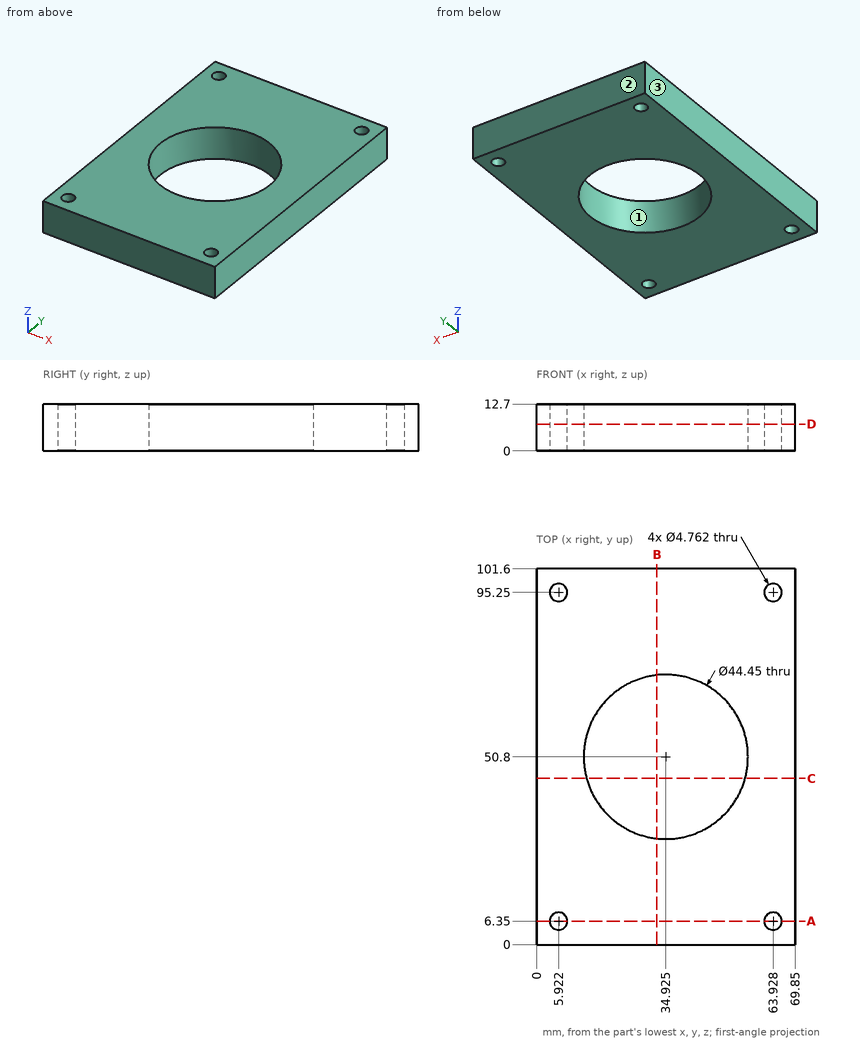
Source: three-view drawing plus pictorial views. Frame: mm from the lowest corner of the part. Coordinates: 2 decimals unless noted, no trailing zeros. Loops run counter-clockwise (first coordinate to the right, second up) from the corner with the lowest first, then second, coordinate; pieces in that order, holes last. Notation, with made-up numbers: (-14, 14.25) -> (14, 14.25) arc R25 cw to (14, 45.25) -> close; hole circle Ø8 at (83, 45). An arc over 180 degrees is marked (long way). One line per item, written item: value.
(1) Ray query, line 1 along Y through (x, z) = (4.5, 6.75); line 2 along Y through (x, z) = (63.5, 5.5); line 3 along Y through (x, z) = (26.5, 10) (1 decimal). Return the intervals inside material, ascending.
Answer below:
line 1: y = 0 to 4.44, 8.26 to 93.34, 97.16 to 101.6
line 2: y = 0 to 4.01, 8.69 to 92.91, 97.59 to 101.6
line 3: y = 0 to 30.2, 71.4 to 101.6
(2) Cut plane C-C (y = 45). Output: boundary loops of the cut face in (x, z), then the cut area to 3 significant figures.
Answer below:
outline: (0, 0) -> (13.47, 0) -> (13.47, 12.7) -> (0, 12.7) -> close; (56.38, 0) -> (69.85, 0) -> (69.85, 12.7) -> (56.38, 12.7) -> close
area: 342 mm2
(3) Cut plane A-A (y = 6.35). Output: boundary loops of the cut face in (x, z), then the cut area to 3 significant figures.
Answer below:
outline: (0, 0) -> (3.54, 0) -> (3.54, 12.7) -> (0, 12.7) -> close; (8.3, 0) -> (61.55, 0) -> (61.55, 12.7) -> (8.3, 12.7) -> close; (66.31, 0) -> (69.85, 0) -> (69.85, 12.7) -> (66.31, 12.7) -> close
area: 766 mm2
(4) Pin query (flat end, axial travel): pin 1 Ø3 at (x, y) = (5.92, 95.25) entering from +Z. Return the tip coordinate at first contact, or that it passes through.
Answer below:
pin 1: passes through
(5) Cut plane B-B (x = 32.5). Output: boundary loops of the cut face in (y, z), then the cut area to 3 significant figures.
Answer below:
outline: (0, 0) -> (28.71, 0) -> (28.71, 12.7) -> (0, 12.7) -> close; (72.89, 0) -> (101.6, 0) -> (101.6, 12.7) -> (72.89, 12.7) -> close
area: 729 mm2
(6) Draft query along Y for the marked faces 1, 2 and 3. Return one class per face: pulls with the +Y half, pulls with the -Y half, needs draft (parallel to the pull), parting line crosses it, or undercut.
Answer below:
face 1: undercut
face 2: pulls with the +Y half
face 3: needs draft
(7) Cut plane D-D (z = 7.25). Give the number of separate pieces and of enclosed holes in the cut face, then the cut area to 3 significant figures.
Answer below:
separate pieces: 1
enclosed holes: 5
area: 5,470 mm2
